The listing builds one solid part. Answer for the finished solid, in the listing's coordinates (mm). Round coordinates to 2 decimals unless told otherwise and drop trailing zeros. Loops run counter-clockwise (first coordinate to the right, second up) from the corner with the lowest first, then second, coordinate; pieces in that order, holes last. Notation, with made-up numbers: (58, 57) - (117, 57) arc R34 cw to (117, 95) - close; hole circle Ø7 at (11.5, 13.25). An arc over 180 degrees is marked (long way). Write item = value, one per line. Start each with the question number.
1) Section A-A, the plane z = 33.5 is taken. Determine the outline of the cut face in (x, y), and give its area (3 significant figures).
2) Straight lines are drawn through the part: line 1 along Y through (x, z) = (121.5, 137.5); line 2 along Y through (x, z) = (119.5, 152); line 3 along Z through (x, y) = (140.5, 285). For each, find the intervals that lie inside material, in ascending order.
3) Given pin 1 Ø2 at (x, z) = (121, 131) entering from +Y; pin 2 Ø10 at (y, z) = (303, 200) entering from -X; pin 3 Ø5 at (y, z) = (282.5, 110) entering from -X, each flat-ended and moving along its own axis, determine where each tip first touches the part or whether it passes through.
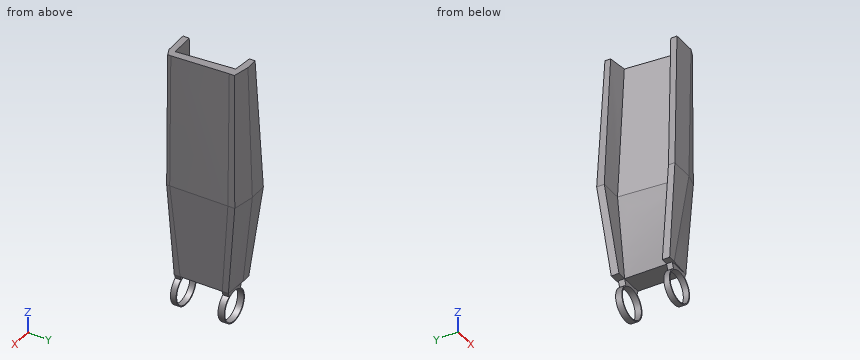
from build123d import *

# Parameters (mm, degrees)
SKETCH4_R           = 13.33935295
BOSS_EXTRUDE1_DEPTH = 5.387848
BOSS_EXTRUDE2_START = -41.145202
SKETCH4_2_R         = 13.33935295
BOSS_EXTRUDE2_DEPTH = 4.89559


with BuildPart() as part:
    # Sketch1 → Loft1 section 0
    with BuildSketch(Plane.XY.offset(238.871252)):
        with BuildLine():
            Line((117.449346, 305.101244), (133.79958, 303.314354))
            Line((133.79958, 303.314354), (138.168888, 253.734316))
            Line((138.168888, 253.734316), (118.163594, 253.574042))
            Line((118.163594, 253.574042), (118.210076, 248.25706))
            Line((118.210076, 248.25706), (138.215116, 248.41708))
            Line((138.215116, 248.41708), (144.422368, 251.041916))
            Line((144.422368, 251.041916), (144.398492, 253.7841))
            Line((144.398492, 253.7841), (141.414246, 302.436784))
            Line((141.414246, 302.436784), (141.376146, 306.803552))
            Line((141.376146, 306.803552), (127.531876, 310.087518))
            Line((127.531876, 310.087518), (117.406674, 310.006492))
            Line((117.406674, 310.006492), (117.449346, 305.101244))
        make_face()
    # Sketch2 → Loft1 section 1
    with BuildSketch(Plane.XY.offset(123.421394)):
        with BuildLine():
            Line((112.248188, 313.980322), (127.943864, 314.106052))
            Line((127.943864, 314.106052), (146.665442, 310.414162))
            Line((146.665442, 310.414162), (146.717258, 304.488342))
            Line((146.717258, 304.488342), (147.153376, 254.497586))
            Line((147.153376, 254.497586), (147.176236, 251.879608))
            Line((147.176236, 251.879608), (136.055354, 248.87809))
            Line((136.055354, 248.87809), (116.05006, 248.717816))
            Line((116.05006, 248.717816), (116.002054, 254.247904))
            Line((116.002054, 254.247904), (136.007094, 254.408178))
            Line((136.007094, 254.408178), (131.213352, 307.596286))
            Line((131.213352, 307.596286), (112.305084, 307.444902))
            Line((112.305084, 307.444902), (112.248188, 313.980322))
        make_face()
    loft()

    # Sketch2<3> → Loft2 section 0
    with BuildSketch(Plane.XY.offset(123.421394)):
        with BuildLine():
            Line((112.248188, 313.980322), (127.943864, 314.106052))
            Line((127.943864, 314.106052), (146.665442, 310.414162))
            Line((146.665442, 310.414162), (146.717258, 304.488342))
            Line((146.717258, 304.488342), (147.153376, 254.497586))
            Line((147.153376, 254.497586), (147.176236, 251.879608))
            Line((147.176236, 251.879608), (136.055354, 248.87809))
            Line((136.055354, 248.87809), (116.05006, 248.717816))
            Line((116.05006, 248.717816), (116.002054, 254.247904))
            Line((116.002054, 254.247904), (136.007094, 254.408178))
            Line((136.007094, 254.408178), (131.213352, 307.596286))
            Line((131.213352, 307.596286), (112.305084, 307.444902))
            Line((112.305084, 307.444902), (112.248188, 313.980322))
        make_face()
    # Sketch3 → Loft2 section 1
    with BuildSketch(Plane.XY.offset(44.31157)):
        with BuildLine():
            Line((119.47779, 299.154342), (119.419878, 305.769518))
            Line((119.419878, 305.769518), (127.526288, 305.834288))
            Line((127.526288, 305.834288), (146.226276, 304.60696))
            Line((146.226276, 304.60696), (146.271996, 299.368972))
            Line((146.271996, 299.368972), (146.588226, 263.119108))
            Line((146.588226, 263.119108), (146.632168, 258.073906))
            Line((146.632168, 258.073906), (127.955548, 256.62763))
            Line((127.955548, 256.62763), (121.519188, 256.576068))
            Line((121.519188, 256.576068), (121.463816, 262.91794))
            Line((121.463816, 262.91794), (127.900176, 262.969502))
            Line((127.900176, 262.969502), (127.583946, 299.219112))
            Line((127.583946, 299.219112), (119.47779, 299.154342))
        make_face()
    loft()

    # Sketch4 → Boss-Extrude1 (add)
    with BuildSketch(Plane(origin=(0, 299.219112, 0), x_dir=(1, 0, 0), z_dir=(0, 1, 0))):
        with BuildLine():
            Line((146.226276, -44.31157), (145.07845, -40.361616))
            ThreePointArc((145.07845, -40.361616), (138.59477889, -14.045079031), (129.276856, -39.496492))
            Line((129.276856, -39.496492), (127.526288, -44.31157))
            Line((127.526288, -44.31157), (146.226276, -44.31157))
        make_face()
        with Locations(Location((137.820198563, -28.192881954, 0), (0, 0, 270))):
            Circle(SKETCH4_R, mode=Mode.SUBTRACT)
    extrude(amount=BOSS_EXTRUDE1_DEPTH)

    # Sketch4<2> → Boss-Extrude2 (add)
    with BuildSketch(Plane(origin=(0, 299.219112, 0), x_dir=(1, 0, 0), z_dir=(0, 1, 0)).offset(BOSS_EXTRUDE2_START)):
        with BuildLine():
            Line((146.226276, -44.31157), (145.07845, -40.361616))
            ThreePointArc((145.07845, -40.361616), (138.59477889, -14.045079031), (129.276856, -39.496492))
            Line((129.276856, -39.496492), (127.526288, -44.31157))
            Line((127.526288, -44.31157), (146.226276, -44.31157))
        make_face()
        with Locations(Location((137.820198563, -28.192881954, 0), (0, 0, 270))):
            Circle(SKETCH4_2_R, mode=Mode.SUBTRACT)
    extrude(amount=BOSS_EXTRUDE2_DEPTH)


solid = part.part
Geometry check:
q1.outline = (124.68, 258.07) - (125.58, 258.07) - (125.58, 262.97) - (124.68, 262.97) - close; (124.68, 299.22) - (125.58, 299.22) - (125.58, 304.61) - (124.68, 304.61) - close; (150.06, 258.07) - (150.96, 258.07) - (150.96, 262.97) - (150.06, 262.97) - close; (150.06, 299.22) - (150.96, 299.22) - (150.96, 304.61) - (150.06, 304.61) - close
q1.area = 18.5 mm2
q2.line_1 = 248.7 to 254.21, 307.12 to 313.56
q2.line_2 = 248.63 to 254.1, 306.76 to 313.04
q2.line_3 = 44.31 to 238.87
q3.pin_1 = 313.82
q3.pin_2 = 115.54
q3.pin_3 = 132.23
